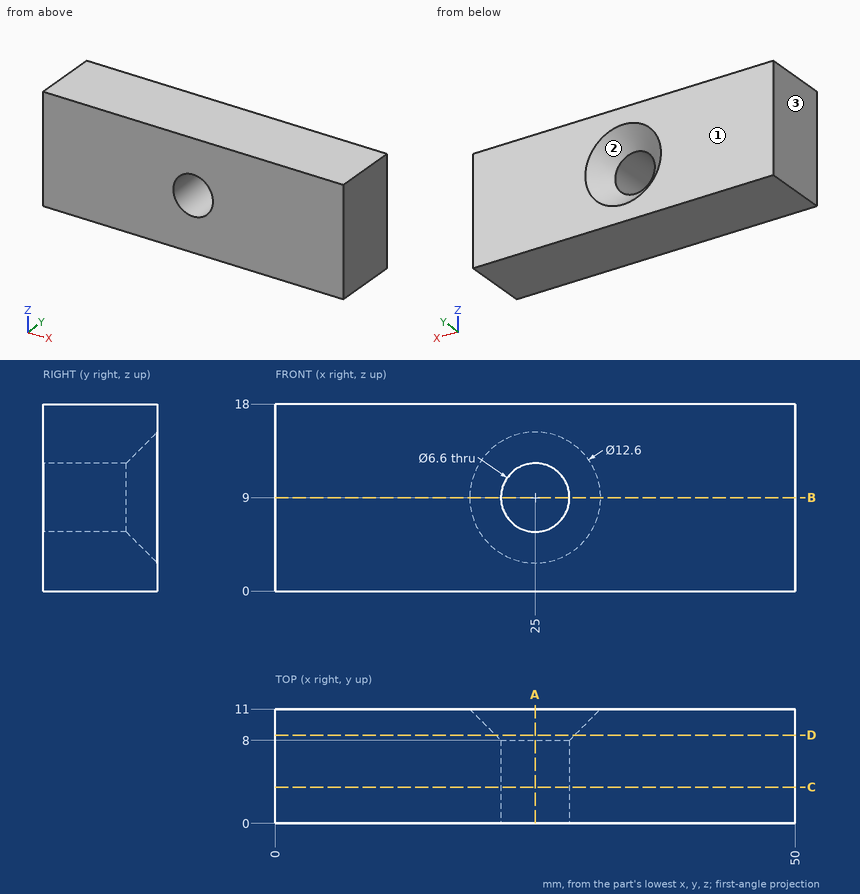
Geometry check sheet. Reference: drawing and pictorial views, mm from the part's lowest x, y, z. Give positions to 0.01 mm unless a question says otherwise; leave off trailing zeros. Order: outer loops, then holes, each group sorted by start corner. A loop starts at its lowest first (then second) coordinate and runs counter-clockwise, first axis right, second up. Notation, with made-up numbers: (80, -37.75) - (129, -37.75) arc R14 ccw to (129, -10.75) - close; hole circle Ø7 at (58.25, 9.25). An arc over 180 degrees is marked (long way). Answer as CSV lines item,"result".
1. Section check A-A (x = 25). Record the boundary of the cut face in (y, z), then the cut area to 3 significant figures.
Result sheet:
outline,"(0, 0) - (11, 0) - (11, 2.7) - (8, 5.7) - (0, 5.7) - close; (0, 12.3) - (8, 12.3) - (11, 15.3) - (11, 18) - (0, 18) - close"
area,"116 mm²"
2. Mould release check, pull along X, two halves, no side actions. Record for the marked faces 1, 2 and 3: released by +X, released by -X, zero draft, split by the parting line, or undercut.
Result sheet:
face 1,"zero draft"
face 2,"undercut"
face 3,"released by -X"
3. Section check D-D (y = 8.5). Record the boundary of the cut face in (x, z), then the cut area to 3 significant figures.
Result sheet:
outline,"(0, 0) - (50, 0) - (50, 18) - (0, 18) - close; hole circle Ø7.6 at (25, 9)"
area,"855 mm²"
4. Scan lines: probe 1 along X at (y, z) = (5.5, 9); probe 2 along Z at (x, y) = (25, 3.5); probe 3 along X at (y, z) = (5.5, 10.75). Record each from-to range of solid material in increasing order. Write a range as from..to.
Result sheet:
probe 1,"0..21.7, 28.3..50"
probe 2,"0..5.7, 12.3..18"
probe 3,"0..22.2, 27.8..50"
5. Go/stop test with a flat-tipped pin: P1, Ø8.5, axis at x = 25, z = 9, coming from the +Y side. Record where the tip stops, or that it passes through.
Result sheet:
P1,"y = 8.95"
6. Section check B-B (z = 9). Record the boundary of the cut face in (x, y), then the cut area to 3 significant figures.
Result sheet:
outline,"(0, 0) - (21.7, 0) - (21.7, 8) - (18.7, 11) - (0, 11) - close; (28.3, 0) - (50, 0) - (50, 11) - (31.3, 11) - (28.3, 8) - close"
area,"468 mm²"
7. Section check C-C (y = 3.5). Record the boundary of the cut face in (x, z).
Result sheet:
outline,"(0, 0) - (50, 0) - (50, 18) - (0, 18) - close; hole circle Ø6.6 at (25, 9)"
